```python
from build123d import *

# Parameters (mm, degrees)
ESQUISSE2_W             = 30
ESQUISSE2_H             = 15
BOSS_EXTRU_1_DEPTH      = 25
ESQUISSE3_W             = 8
ESQUISSE3_H             = 15
BOSS_EXTRU_2_DEPTH      = 11
ENL_V_MAT_EXTRU_1_REACH = 17
ESQUISSE4_R             = 2.5
ENL_V_MAT_EXTRU_2_REACH = 10
ESQUISSE7_W             = 50
ESQUISSE7_H             = 15
ESQUISSE7_R             = 2.1
BOSS_EXTRU_4_DEPTH      = 5
CONG_2_R                = 4


with BuildPart() as part:
    # Esquisse2 → Boss.-Extru.1 (new body)
    with BuildSketch(Plane(origin=(0, 0, 0), x_dir=(1, 0, 0), z_dir=(0, 1, 0))):
        Rectangle(ESQUISSE2_W, ESQUISSE2_H)
    extrude(amount=BOSS_EXTRU_1_DEPTH)

    # Esquisse3 → Boss.-Extru.2 (add)
    with BuildSketch(Plane(origin=(0, 25, 0), x_dir=(1, 0, 0), z_dir=(0, 1, 0))):
        with Locations((11, 0)):
            Rectangle(ESQUISSE3_W, ESQUISSE3_H)
    extrude(amount=BOSS_EXTRU_2_DEPTH)

    # Esquisse4 → Enlèv. mat.-Extru.1 (cut, up to next)
    with BuildSketch(Plane.XY.offset(7.5), mode=Mode.PRIVATE) as enl_v_mat_extru_1_sk1:
        with Locations((-4, 15)):
            Circle(ESQUISSE4_R)
    enl_v_mat_extru_1_tool1 = extrude(enl_v_mat_extru_1_sk1.sketch, amount=-ENL_V_MAT_EXTRU_1_REACH, mode=Mode.PRIVATE) & part.part
    add(enl_v_mat_extru_1_tool1.solids().sort_by_distance((-4, 15, 7.5))[0], mode=Mode.SUBTRACT)

    # Esquisse5 → Enlèv. mat.-Extru.2 (cut, up to next)
    with BuildSketch(Plane.ZY.offset(-7), mode=Mode.PRIVATE) as enl_v_mat_extru_2_sk1:
        with BuildLine():
            Line((5.75, 33), (5.75, 28))
            ThreePointArc((5.75, 28), (4.5, 26.75), (3.25, 28))
            Line((3.25, 28), (3.25, 33))
            ThreePointArc((3.25, 33), (4.5, 34.25), (5.75, 33))
        make_face()
    enl_v_mat_extru_2_tool1 = extrude(enl_v_mat_extru_2_sk1.sketch, amount=-ENL_V_MAT_EXTRU_2_REACH, mode=Mode.PRIVATE) & part.part
    add(enl_v_mat_extru_2_tool1.solids().sort_by_distance((7, 30.5, 4.5))[0], mode=Mode.SUBTRACT)
    # Esquisse5 → Enlèv. mat.-Extru.2 (cut, up to next)
    with BuildSketch(Plane.ZY.offset(-7), mode=Mode.PRIVATE) as enl_v_mat_extru_2_sk2:
        with BuildLine():
            Line((-3.25, 33), (-3.25, 28))
            ThreePointArc((-3.25, 28), (-4.5, 26.75), (-5.75, 28))
            Line((-5.75, 28), (-5.75, 33))
            ThreePointArc((-5.75, 33), (-4.5, 34.25), (-3.25, 33))
        make_face()
    enl_v_mat_extru_2_tool2 = extrude(enl_v_mat_extru_2_sk2.sketch, amount=-ENL_V_MAT_EXTRU_2_REACH, mode=Mode.PRIVATE) & part.part
    add(enl_v_mat_extru_2_tool2.solids().sort_by_distance((7, 30.5, -4.5))[0], mode=Mode.SUBTRACT)

    # Esquisse7 → Boss.-Extru.4 (add)
    with BuildSketch(Plane.XZ):
        Rectangle(ESQUISSE7_W, ESQUISSE7_H)
        with Locations((20, 0)):
            Circle(ESQUISSE7_R, mode=Mode.SUBTRACT)
        with Locations((-20, 0)):
            Circle(ESQUISSE7_R, mode=Mode.SUBTRACT)
    extrude(amount=-BOSS_EXTRU_4_DEPTH)

    # Congé2
    cong_2_edges = [part.edges().sort_by_distance(p)[0] for p in [
        (25, 2.5, -7.5),
        (-25, 2.5, 7.5),
        (25, 2.5, 7.5),
        (-25, 2.5, -7.5),
    ]]
    fillet(cong_2_edges, radius=CONG_2_R)


solid = part.part
```
Build history of the part. All positions in model axes, mm. A direction names the side the tool comes from. Coordinates: 2 decimals unless noted, no trailing zeros. Order: outer loops, then holes, each group sorted by start corner. A loop starts at its lowest first (then second) coordinate and runs counter-clockwise, first axis right, second up. Notation, with made-up numbers: (35, 48.5) -> (47, 48.5) arc R30 ccw to (47, 73.5) -> close; hole circle Ø7 at (42.5, 75.5). An arc over 180 degrees is marked (long way). Answer in a Markdown table with one row per item. Add a question column.
Q1. Band-saw the part on D-D, the plane z = -4.5. List the corners of the cut face in (x, y), then the cut area to 3 significant figures.
Q2. Band-saw the part on A-A, the plane z = 0. List the corners of the cut face in (x, y), then the cut area to 3 significant figures.
Q3. Wall check: line 1 along Z through (x, y) = (12, 28); line 2 along Z through (x, y) = (-20, 2.15); line 3 along X through (y, z) = (28, -1.25). Give the ranges that are in metal, low to high. Write a range as [from, to].
Q4. Band-saw the part on B-B, the plane y = 15. List the corners of the cut face in (x, z).
Q5. Mould opens along Z. For faces 6 (the face through (0, 14, 7.5)), 7 (the face through (-4, 25, 0)), 8 (the face through (11, 30, -5.75)) say: +Z half, -Z half, draft (parallel to the pull), parting line (faces both ways), or undercut.
Q6. Band-saw the part on C-C, the plane x = -20. List the corners of the cut face in (y, z), then the cut area to 3 significant figures.
Q7. Drop flat-ended pins along their axis: pin 1 (2 mm diameter, centred on x = -12.5, y = 26.5, fed in from +Z); pin 2 (9 mm diameter, centred on y = 31.5, z = -1, fed in from -X); pin 3 (7.5 mm diameter, centred on y = 14.5, z = -0.5, fed in from +X); pin 4 (3 mm diameter, centred on y = 21, z = 5.5, fed in from -X). Give the stop position or say it passes through.
Q8. Which spindle directions (+Z, -Z, +X, -X, +Y, -Y) get a long thin tool onto all of the face, cutting with end or side? Do faces 1 (the face through (17.7, 5, 0.1)), 2 (the face through (7, 30, 0)), 3 (the face through (11, 30, 3.25)), 4 (the face through (-25, 2, 0)), 5 (the face through (0, 14, -7.5)). Say none if no direction does.
Answers follow:
| question | item | result |
|---|---|---|
| 1 | outline | (-24.87, 0) -> (24.87, 0) -> (24.87, 5) -> (15, 5) -> (15, 26.75) -> (7, 26.75) -> (7, 25) -> (-15, 25) -> (-15, 5) -> (-24.87, 5) -> close; (7, 34.25) -> (15, 34.25) -> (15, 36) -> (7, 36) -> close; hole circle Ø5 at (-4, 15) |
| 1 | area | 857 mm^2 |
| 2 | outline | (-25, 0) -> (-22.1, 0) -> (-22.1, 5) -> (-25, 5) -> close; (-17.9, 0) -> (17.9, 0) -> (17.9, 5) -> (15, 5) -> (15, 36) -> (7, 36) -> (7, 25) -> (-15, 25) -> (-15, 5) -> (-17.9, 5) -> close; (22.1, 0) -> (25, 0) -> (25, 5) -> (22.1, 5) -> close; hole circle Ø5 at (-4, 15) |
| 2 | area | 876 mm^2 |
| 3 | line 1 | [-7.5, -5.75], [-3.25, 3.25], [5.75, 7.5] |
| 3 | line 2 | [-7.5, -2.1], [2.1, 7.5] |
| 3 | line 3 | [7, 15] |
| 4 | outline | (-15, -7.5) -> (-6.5, -7.5) -> (-6.5, 7.5) -> (-15, 7.5) -> close; (-1.5, -7.5) -> (15, -7.5) -> (15, 7.5) -> (-1.5, 7.5) -> close |
| 5 | face 6 | +Z half |
| 5 | face 7 | draft |
| 5 | face 8 | undercut |
| 6 | outline | (0, -7.5) -> (5, -7.5) -> (5, -2.1) -> (0, -2.1) -> close; (0, 2.1) -> (5, 2.1) -> (5, 7.5) -> (0, 7.5) -> close |
| 6 | area | 54.0 mm^2 |
| 7 | pin 1 | through |
| 7 | pin 2 | x = 7 |
| 7 | pin 3 | x = 15 |
| 7 | pin 4 | x = -15 |
| 8 | face 1 | +Z, -Z, +X, +Y |
| 8 | face 2 | +Z, -Z, -X, +Y |
| 8 | face 3 | +X, -X |
| 8 | face 4 | +Z, -Z, -X, +Y, -Y |
| 8 | face 5 | -Z, +X, -X, +Y, -Y |
